```python
from build123d import *

# Parameters (mm, degrees)
F0_W     = 210
F0_H     = 50
F1_DEPTH = 10
F3_DEPTH = 10.001
F4_SIZE  = 2


with BuildPart() as f1:
    # F0 (on Top) → F1 (new body)
    with BuildSketch(Plane.XY):
        Rectangle(F0_W, F0_H)
    extrude(amount=F1_DEPTH)

    # F2 (on face) → F3 (cut, through all)
    with BuildSketch(Plane.XY.offset(10)):
        with BuildLine():
            ThreePointArc((-88, -5), (-90, -3), (-92, -5))
            Line((-92, -5), (-88, -5))
        make_face()
        with BuildLine():
            Line((-88, -5), (-92, -5))
            ThreePointArc((-92, -5), (-90, -7), (-88, -5))
        make_face()
        with BuildLine():
            ThreePointArc((-58, -5), (-60, -3), (-62, -5))
            Line((-62, -5), (-58, -5))
        make_face()
        with BuildLine():
            Line((-58, -5), (-62, -5))
            ThreePointArc((-62, -5), (-60, -7), (-58, -5))
        make_face()
        with BuildLine():
            ThreePointArc((-28, -5), (-30, -3), (-32, -5))
            Line((-32, -5), (-28, -5))
        make_face()
        with BuildLine():
            Line((-28, -5), (-32, -5))
            ThreePointArc((-32, -5), (-30, -7), (-28, -5))
        make_face()
        with BuildLine():
            ThreePointArc((32, -5), (30, -3), (28, -5))
            Line((28, -5), (32, -5))
        make_face()
        with BuildLine():
            Line((32, -5), (28, -5))
            ThreePointArc((28, -5), (30, -7), (32, -5))
        make_face()
        with BuildLine():
            ThreePointArc((62, -5), (60, -3), (58, -5))
            Line((58, -5), (62, -5))
        make_face()
        with BuildLine():
            Line((62, -5), (58, -5))
            ThreePointArc((58, -5), (60, -7), (62, -5))
        make_face()
        with BuildLine():
            Line((88, -5), (92, -5))
            ThreePointArc((92, -5), (90, -3), (88, -5))
        make_face()
        with BuildLine():
            ThreePointArc((88, -5), (90, -7), (92, -5))
            Line((92, -5), (88, -5))
        make_face()
    extrude(amount=-F3_DEPTH, mode=Mode.SUBTRACT)

    # F4
    f4_edges = [f1.edges().sort_by_distance(p)[0] for p in [
        (-88, -5, 10),
        (-58, -5, 10),
        (-28, -5, 10),
        (32, -5, 10),
        (62, -5, 10),
        (92, -5, 10),
    ]]
    chamfer(f4_edges, length=F4_SIZE)


solid = f1.part
```
Geometry check sheet. Reference: the model listing, model coordinates, mm. Coordinates: 2 decimals unless noted, no trailing zeros. Order: outer loops, then holes, each group sorted by start corner. A loop starts at its lowest first (then second) coordinate and runs counter-clockwise, first axis right, second up.
Item 1: Section check A-A (x = 90). Enter the section's corners in (y, z).
Item 2: Mould release check, pull along Y, two halves, no side actions. Record for faces 1 (the flat face through (-1, 0, 0)), 2 (the cylindrical face through (-58, -5, 4)), 3 (the flat face through (-1, -25, 5)): released by +Y, released by -Y, zero draft, split by the parting line, or undercut.
Item 3: Scan line: line 1 along Y through (x, z) = (30, 6). Record every from-to range of solid material in increasing order.
Check sheet entries:
1. outline: (-25, 0) - (-7, 0) - (-7, 8) - (-9, 10) - (-25, 10) - close; (-3, 0) - (25, 0) - (25, 10) - (-1, 10) - (-3, 8) - close
2. face 1: zero draft
2. face 2: undercut
2. face 3: released by -Y
3. line 1: y = -25 to -7, -3 to 25
